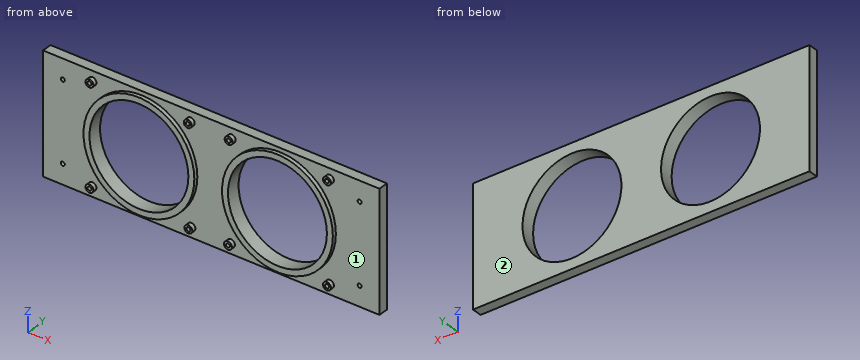
```python
from build123d import *

# Parameters (mm, degrees)
F0_W     = 170.0022
F0_H     = 60
F0_R     = 2
F0_R_2   = 1
F0_R_3   = 28
F0_R_4   = 25
F1_DEPTH = 5
F2_DEPTH = 7
F3_DEPTH = 3
F4_DEPTH = 7
F5_START = 2
F5_DEPTH = 3


with BuildPart() as f1:
    # F0 (on Front) → F1 (new body)
    with BuildSketch(Plane.XZ):
        with Locations((63.8357337121, -49.967572093)):
            Rectangle(F0_W, F0_H)
        with Locations((3.8346337121, -74.967572093)):
            Circle(F0_R, mode=Mode.SUBTRACT)
        with Locations((-11.1653662879, -69.967572093)):
            Circle(F0_R_2, mode=Mode.SUBTRACT)
        with Locations((53.8346337121, -74.967572093)):
            Circle(F0_R, mode=Mode.SUBTRACT)
        with Locations((73.8368337121, -74.967572093)):
            Circle(F0_R, mode=Mode.SUBTRACT)
        with Locations((123.8368337121, -74.967572093)):
            Circle(F0_R, mode=Mode.SUBTRACT)
        with Locations((138.8368337121, -69.967572093)):
            Circle(F0_R_2, mode=Mode.SUBTRACT)
        with Locations((98.8368337121, -49.967572093)):
            Circle(F0_R_3, mode=Mode.SUBTRACT)
        with Locations((28.8346337121, -49.967572093)):
            Circle(F0_R_3, mode=Mode.SUBTRACT)
        with Locations((-11.1653662879, -29.967572093)):
            Circle(F0_R_2, mode=Mode.SUBTRACT)
        with Locations((3.8346337121, -24.967572093)):
            Circle(F0_R, mode=Mode.SUBTRACT)
        with Locations((53.4981064092, -24.967572093)):
            Circle(F0_R, mode=Mode.SUBTRACT)
        with Locations((74.1733610149, -24.967572093)):
            Circle(F0_R, mode=Mode.SUBTRACT)
        with Locations((138.8368337121, -29.967572093)):
            Circle(F0_R_2, mode=Mode.SUBTRACT)
        with Locations((123.8368337121, -24.967572093)):
            Circle(F0_R, mode=Mode.SUBTRACT)
        with Locations((28.8346337121, -49.967572093)):
            Circle(F0_R_3)
        with Locations((28.8346337121, -49.967572093)):
            Circle(F0_R_4, mode=Mode.SUBTRACT)
        with Locations((98.8368337121, -49.967572093)):
            Circle(F0_R_3)
        with Locations((98.8368337121, -49.967572093)):
            Circle(F0_R_4, mode=Mode.SUBTRACT)
        with Locations((3.8346337121, -74.967572093)):
            Circle(F0_R)
        with Locations((3.8346337121, -74.967572093)):
            Circle(F0_R_2, mode=Mode.SUBTRACT)
        with Locations((53.8346337121, -74.967572093)):
            Circle(F0_R)
        with Locations((53.8346337121, -74.967572093)):
            Circle(F0_R_2, mode=Mode.SUBTRACT)
        with Locations((73.8368337121, -74.967572093)):
            Circle(F0_R)
        with Locations((73.8368337121, -74.967572093)):
            Circle(F0_R_2, mode=Mode.SUBTRACT)
        with Locations((123.8368337121, -74.967572093)):
            Circle(F0_R)
        with Locations((123.8368337121, -74.967572093)):
            Circle(F0_R_2, mode=Mode.SUBTRACT)
        with Locations((123.8368337121, -24.967572093)):
            Circle(F0_R)
        with Locations((123.8368337121, -24.967572093)):
            Circle(F0_R_2, mode=Mode.SUBTRACT)
        with Locations((74.1733610149, -24.967572093)):
            Circle(F0_R)
        with Locations((74.1733610149, -24.967572093)):
            Circle(F0_R_2, mode=Mode.SUBTRACT)
        with Locations((53.4981064092, -24.967572093)):
            Circle(F0_R)
        with Locations((53.4981064092, -24.967572093)):
            Circle(F0_R_2, mode=Mode.SUBTRACT)
        with Locations((3.8346337121, -24.967572093)):
            Circle(F0_R)
        with Locations((3.8346337121, -24.967572093)):
            Circle(F0_R_2, mode=Mode.SUBTRACT)
        with Locations((-11.1653662879, -69.967572093)):
            Circle(F0_R_2)
        with Locations((3.8346337121, -74.967572093)):
            Circle(F0_R_2)
        with Locations((53.8346337121, -74.967572093)):
            Circle(F0_R_2)
        with Locations((73.8368337121, -74.967572093)):
            Circle(F0_R_2)
        with Locations((123.8368337121, -74.967572093)):
            Circle(F0_R_2)
        with Locations((138.8368337121, -69.967572093)):
            Circle(F0_R_2)
        with Locations((138.8368337121, -29.967572093)):
            Circle(F0_R_2)
        with Locations((123.8368337121, -24.967572093)):
            Circle(F0_R_2)
        with Locations((74.1733610149, -24.967572093)):
            Circle(F0_R_2)
        with Locations((53.4981064092, -24.967572093)):
            Circle(F0_R_2)
        with Locations((3.8346337121, -24.967572093)):
            Circle(F0_R_2)
        with Locations((-11.1653662879, -29.967572093)):
            Circle(F0_R_2)
    extrude(amount=F1_DEPTH)

    # F0 (on Front) → F2 (join)
    with BuildSketch(Plane.XZ):
        with Locations((3.8346337121, -24.967572093)):
            Circle(F0_R)
        with Locations((3.8346337121, -24.967572093)):
            Circle(F0_R_2, mode=Mode.SUBTRACT)
        with Locations((53.4981064092, -24.967572093)):
            Circle(F0_R)
        with Locations((53.4981064092, -24.967572093)):
            Circle(F0_R_2, mode=Mode.SUBTRACT)
        with Locations((74.1733610149, -24.967572093)):
            Circle(F0_R)
        with Locations((74.1733610149, -24.967572093)):
            Circle(F0_R_2, mode=Mode.SUBTRACT)
        with Locations((123.8368337121, -24.967572093)):
            Circle(F0_R)
        with Locations((123.8368337121, -24.967572093)):
            Circle(F0_R_2, mode=Mode.SUBTRACT)
        with Locations((123.8368337121, -74.967572093)):
            Circle(F0_R)
        with Locations((123.8368337121, -74.967572093)):
            Circle(F0_R_2, mode=Mode.SUBTRACT)
        with Locations((73.8368337121, -74.967572093)):
            Circle(F0_R)
        with Locations((73.8368337121, -74.967572093)):
            Circle(F0_R_2, mode=Mode.SUBTRACT)
        with Locations((53.8346337121, -74.967572093)):
            Circle(F0_R)
        with Locations((53.8346337121, -74.967572093)):
            Circle(F0_R_2, mode=Mode.SUBTRACT)
        with Locations((3.8346337121, -74.967572093)):
            Circle(F0_R)
        with Locations((3.8346337121, -74.967572093)):
            Circle(F0_R_2, mode=Mode.SUBTRACT)
    extrude(amount=F2_DEPTH)

    # F3 (cut): faces of the model
    f3_faces = [f1.faces().sort_by_distance(p)[0] for p in [
        (53.8346337121, -5, -74.967572093),
        (73.8368337121, -5, -74.967572093),
        (3.8346337121, -5, -74.967572093),
        (3.8346337121, -5, -24.967572093),
        (53.4981064092, -5, -24.967572093),
        (74.1733610149, -5, -24.967572093),
        (123.8368337121, -5, -24.967572093),
        (123.8368337121, -5, -74.967572093),
    ]]
    extrude(f3_faces, amount=-F3_DEPTH, mode=Mode.SUBTRACT)

    # F0 (on Front) → F4 (join)
    with BuildSketch(Plane.XZ):
        with Locations((98.8368337121, -49.967572093)):
            Circle(F0_R_3)
        with Locations((98.8368337121, -49.967572093)):
            Circle(F0_R_4, mode=Mode.SUBTRACT)
        with Locations((28.8346337121, -49.967572093)):
            Circle(F0_R_3)
        with Locations((28.8346337121, -49.967572093)):
            Circle(F0_R_4, mode=Mode.SUBTRACT)
    extrude(amount=F4_DEPTH)

    # F0 (on Front) → F5 (cut)
    with BuildSketch(Plane.XZ.offset(F5_START)):
        with Locations((-11.1653662879, -29.967572093)):
            Circle(F0_R_2)
        with Locations((138.8368337121, -29.967572093)):
            Circle(F0_R_2)
        with Locations((138.8368337121, -69.967572093)):
            Circle(F0_R_2)
        with Locations((-11.1653662879, -69.967572093)):
            Circle(F0_R_2)
    extrude(amount=F5_DEPTH, mode=Mode.SUBTRACT)


solid = f1.part
```
Work out the finished part from the listing and answer in its coordinate system (mm). Face numbers are marked on the shaded views. A direction names the side the tool comes from. Coordinates: 2 decimals unless noted, no trailing zeros. Order: outer loops, then holes, each group sorted by start corner. A loop starts at its lowest first (then second) coordinate and runs counter-clockwise, first axis right, second up. Notation, with made-up numbers: M 78.5,65.5 L 120.5,65.5 A13 ccw 120.5,86.5 Z; hole C -25,43 d11. An arc over 180 degrees is marked long. Use CSV: the item, a comma, the result in double quotes.
1) Flat-ended cylindrical pins translate along their axes: pin 1 Ø0.6 at (x, z) = (123.5, -75) entering from -Y; pin 2 Ø10 at (x, z) = (46.5, -73) entering from -Y; pin 3 Ø1.6 at (x, z) = (-11.5, -70) entering from -Y. Find the tip coordinate at first contact, or state that the pin passes through.
Worked out:
pin 1,"stops at y = -2"
pin 2,"stops at y = -7"
pin 3,"stops at y = -5"
2) Section B-B on z = -64 is taken. Write down the section's boundary in (x, y) (3 decimals).
Worked out:
outline,"M -21.165,-5 L 4.605,-5 L 4.605,-7 L 8.144,-7 L 8.144,0 L -21.165,0 Z; M 49.525,-7 L 53.065,-7 L 53.065,-5 L 74.607,-5 L 74.607,-7 L 78.146,-7 L 78.146,0 L 49.525,0 Z; M 119.527,-7 L 123.067,-7 L 123.067,-5 L 148.837,-5 L 148.837,0 L 119.527,0 Z"
3) Section C-C on x = 114.5 is taken. Write down the section's boundary in (y, z), plus the area to 3 significant figures.
Worked out:
outline,"M -7,-73.18 L -5,-73.18 L -5,-79.97 L 0,-79.97 L 0,-69.45 L -7,-69.45 Z; M -7,-30.48 L 0,-30.48 L 0,-19.97 L -5,-19.97 L -5,-26.76 L -7,-26.76 Z"
area,"120 mm^2"
4) For the marked faces 1 and 2, determine the directions among +Z, -Z, +X, -X, +Y, -Y from which every point of the face is accessible in a straight line to the end or side of a thin tool.
Worked out:
face 1,"-Y"
face 2,"+Z, -Z, +X, -X, +Y"
5) Section A-A on x = 96 is taken. Write down the section's boundary in (y, z), plus the area to 3 significant figures.
Worked out:
outline,"M -7,-77.82 L -5,-77.82 L -5,-79.97 L 0,-79.97 L 0,-74.81 L -7,-74.81 Z; M -7,-25.13 L 0,-25.13 L 0,-19.97 L -5,-19.97 L -5,-22.11 L -7,-22.11 Z"
area,"63.7 mm^2"
6) Section D-D on z = -54 is taken. Write down the section's boundary in (x, y), plus the area to 3 significant figures.
Worked out:
outline,"M -21.17,-5 L 1.13,-5 L 1.13,-7 L 4.16,-7 L 4.16,0 L -21.17,0 Z; M 53.51,-7 L 56.54,-7 L 56.54,-5 L 71.13,-5 L 71.13,-7 L 74.16,-7 L 74.16,0 L 53.51,0 Z; M 123.51,-7 L 126.54,-7 L 126.54,-5 L 148.84,-5 L 148.84,0 L 123.51,0 Z"
area,"381 mm^2"
7) Consider line 1 (X direction, y = -5.5, z = -49); line 2 (X direction, y = -0.75, z = -51); line 3 (X direction, y = -0.75, z = -70.5). Determine where each line is inside the solid, lowest interval first. Write a range as [from, to].
Worked out:
line 1,"x = [0.85, 3.85], [53.82, 56.82], [70.85, 73.86], [123.82, 126.82]"
line 2,"x = [-21.17, 3.86], [53.81, 73.86], [123.82, 148.84]"
line 3,"x = [-21.17, 14.57], [43.1, 84.57], [113.1, 148.84]"
